The listing builds one solid part. Answer for the finished solid, in the listing's coordinates (mm). Face numbers are marked on the shaded views. A direction names the side the tool comes from. Coordinates: 2 decimals unless noted, no trailing zeros. Order: outer loops, then holes, each group sorted by start corner. A loop starts at its lowest first (then second) coordinate and runs counter-clockwise, first axis right, second up. Notation, with made-up numbers: M 38.5,21.5 L 83.5,21.5 A18 ccw 83.5,25.5 Z; hole C -40,-18 d8. An arc over 180 degrees is marked long. One line per item, written item: value. Start each with the question number.
Q1. The part is cut by section A-A on x = 0. Give the vertices of the cut face in (y, z).
Q2. For the marked faces 4, 5, 6, 7 and 8, determine the directions among +Z, -Z, +X, -X, +Y, -Y from which every point of the face is accessible in a straight line to the end or side of a thin tool.
Q3. Each of these flat-tipped pins is pushed along its axis until it touches: pin 1 Ø16.5 at (x, z) = (-16, 68) entering from +Y; pin 2 Ø2 at (x, y) = (12.5, -9) entering from +Z; pin 3 Ø0.9 at (x, y) = (14.5, -1) entering from +Z. Where does it stop, or does it pass through?
Q4. The part is cut by section C-C on z = 70.9. Give the number of separate pieces and of enclosed holes in the cut face, then the cut area to 3 significant figures.
Q5. Straight lines are drawn through the part: line 1 along Y through (x, z) = (-7.5, 72); line 2 along Y through (x, z) = (0, 67.75); line 3 along X through (y, z) = (3, 70). For each, find the intervals that lie inside material, in ascending order. Write a range as [from, to].
Q6. The part is cut by section B-B on z = 31. Give the vertices of the cut face in (x, y), then the cut area to 3 significant figures.
Q7. Determine the mould class of the marked faces 1, 2 and 3 for opening direction X: pulls with the +X half, pulls with the -X half, needs draft (parallel to the pull), parting line crosses it, or undercut.
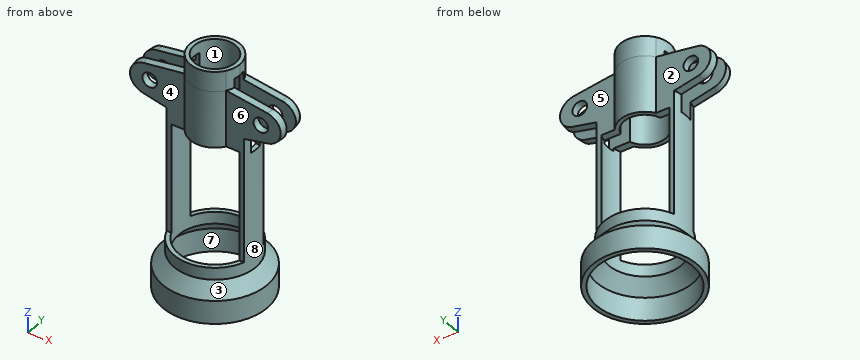
```python
from build123d import *
from build123d import SkipClean  # not in build123d's __all__

# Parameters (mm, degrees)
F3_DEPTH = 68.1
F4_W     = 4.8
F4_H     = 25
F5_DEPTH = 41.80857
F6_R     = 2.65
F7_DEPTH = 25


with BuildPart() as f1:
    # F0 (on Front) → F1 (revolve)
    with BuildSketch(Plane.XZ):
        with BuildLine():
            Line((17.45, 8.5), (17.45, 0))
            Line((17.45, 0), (19.05, 0))
            Line((19.05, 0), (19.05, 8.5))
            Line((19.05, 8.5), (14.9, 13.3))
            Line((14.9, 13.3), (14.9, 63.3))
            Line((14.9, 63.3), (23.2882495839, 65.2334026039))
            ThreePointArc((23.2882495839, 65.2334026039), (27.6657550526, 70.9379230726), (22.8977616622, 76.3203339576))
            Line((22.8977616622, 76.3203339576), (9.05, 78.5))
            Line((9.05, 78.5), (9.05, 85.8))
            Line((9.05, 85.8), (7.55, 85.8))
            Line((7.55, 85.8), (7.55, 57.8))
            Line((7.55, 57.8), (13.3, 57.8))
            Line((13.3, 57.8), (13.3, 13.3))
            Line((13.3, 13.3), (17.45, 8.5))
        make_face()
    revolve(axis=Axis((0, 0, 43.5625389218), (0, 0, 1)))

    # F2 (on face) → F3 (cut)
    with BuildSketch(Plane.XY.offset(85.8)):
        with BuildLine():
            ThreePointArc((7.4761286773, -5.1), (0, -9.05), (-7.4761286773, -5.1))
            Line((-7.4761286773, -5.1), (-33.3200879395, -5.1))
            Line((-33.3200879395, -5.1), (-33.3200879395, -32.3637121379))
            Line((-33.3200879395, -32.3637121379), (33.8455328711, -32.3637121379))
            Line((33.8455328711, -32.3637121379), (33.8455328711, -5.1))
            Line((33.8455328711, -5.1), (7.4761286773, -5.1))
        make_face()
        with BuildLine():
            Line((7.4761286773, 5.1), (33.8455328711, 5.1))
            Line((33.8455328711, 5.1), (33.8455328711, 32.3637121379))
            Line((33.8455328711, 32.3637121379), (-33.3200879395, 32.3637121379))
            Line((-33.3200879395, 32.3637121379), (-33.3200879395, 5.1))
            Line((-33.3200879395, 5.1), (-7.4761286773, 5.1))
            ThreePointArc((-7.4761286773, 5.1), (0, 9.05), (7.4761286773, 5.1))
        make_face()
    with SkipClean():  # cleaning this boolean's faces spoils the solid; the shape is the same uncleaned
        extrude(amount=-F3_DEPTH, mode=Mode.SUBTRACT)

    # F4 (on Right) → F5 (cut, symmetric)
    with BuildSketch(Plane.YZ):
        with Locations((-0.0327096786, 69.3)):
            Rectangle(F4_W, F4_H)
    extrude(amount=F5_DEPTH, both=True, mode=Mode.SUBTRACT)

    # F6 (on face) → F7 (cut)
    with BuildSketch(Plane(origin=(0, 5.1, 0), x_dir=(-1, 0, 0), z_dir=(0, 1, 0))):
        with Locations((-20.0461286773, 70.9)):
            Circle(F6_R)
        with Locations((20.0461286773, 70.9)):
            Circle(F6_R)
    extrude(amount=-F7_DEPTH, mode=Mode.SUBTRACT)


solid = f1.part
```
Output:
1. outline: M -19.05,0 L -17.45,0 L -17.45,8.5 L -13.3,13.3 L -13.3,17.7 L -14.9,17.7 L -14.9,13.3 L -19.05,8.5 Z; M -9.05,57.8 L -7.55,57.8 L -7.55,85.8 L -9.05,85.8 Z; M 7.55,57.8 L 9.05,57.8 L 9.05,85.8 L 7.55,85.8 Z; M 13.3,13.3 L 17.45,8.5 L 17.45,0 L 19.05,0 L 19.05,8.5 L 14.9,13.3 L 14.9,17.7 L 13.3,17.7 Z
2. face 4: +Z, -X, -Y
2. face 5: +Z, +X, +Y
2. face 6: +Z, +X, -Y
2. face 7: -Z
2. face 8: none
3. pin 1: stops at y = 5.1
3. pin 2: stops at z = 17.7
3. pin 3: stops at z = 56.8
4. separate pieces: 6
4. enclosed holes: 0
4. area: 214 mm^2
5. line 1: y = [-5.1, -2.43], [2.37, 5.1]
5. line 2: y = [-9.05, -7.55], [7.55, 9.05]
5. line 3: x = [-27.46, -22.54], [-17.55, -6.93], [6.93, 17.55], [22.54, 27.46]
6. outline: M -14,-5.1 L -12.28,-5.1 A13.3 cw -12.28,5.1 L -14,5.1 A14.9 ccw Z; M 12.28,-5.1 L 14,-5.1 A14.9 ccw 14,5.1 L 12.28,5.1 A13.3 cw Z
6. area: 33.4 mm^2
7. face 1: undercut
7. face 2: needs draft
7. face 3: parting line crosses it
